Work out the finished part from the listing and answer in its coordinate system (mm). A direction names the side the tool comes from. Round coordinates to 2 decimals unless told otherwise and drop trailing zeros. Write each loop counter-clockwise with the first axis right and the second up, starting at its lowest first coordinate (ties: lowest second). Pieces come first, ordered by that corner, then holes. Notation, with made-up numbers: M 39.5,-28.75 L 51.5,-28.75 A17 cw 51.5,-13.75 Z; hole C 82,43 d4. An arc over 180 degrees is marked long. Answer in a Markdown table with one row per item.
Autodesk Inventor part; units mm, degrees
ref_plane "YZ Plane" through (0, 0, 0) normal (1, 0, 0) x (0, 1, 0)
ref_plane "XZ Plane" through (0, 0, 0) normal (0, 1, 0) x (-1, 0, 0)
ref_plane "XY Plane" through (0, 0, 0) normal (0, 0, 1) x (1, 0, 0)
sketch "Skizze1" plane through (0, 0, 0) normal (0, 1, 0) x (-1, 0, 0)
  line L0 (0, 0) -> (13.65, 0) construction
  line L1 (15.3, 9.35) -> (0, 9.35)
  line L2 (3.6, 5) -> (15.3, 5)
  line L3 (15.3, 5) -> (15.3, 9.35)
  line L4 (0, 9.35) -> (3.95, 9.35)
  line L5 (3.6, 5) -> (3.6, -5)
  line L6 (3.95, -9.35) -> (0, -9.35)
  line L7 (0, -9.35) -> (0, 9.35)
  line L8 (0, -9.35) -> (15.3, -9.35)
  line L9 (15.3, -9.35) -> (15.3, -5)
  line L10 (15.3, -5) -> (3.6, -5)
  dimension "d0" = 18.7
  dimension "d1" = 10
  dimension "d2" = 15.3
  dimension "d3" = 3.6
extrude "Extrusion1" add sketch "Skizze1" along normal blind 5
sketch "Skizze3" plane through (0, 0, 0) normal (1, 0, 0) x (0, 1, 0)
  line L0 (0, 9.35) -> (0, -9.35)
  line L1 (0, -9.35) -> (5, -9.35)
  line L2 (5, 9.35) -> (5, -9.35)
  line L3 (0, 9.35) -> (5, 9.35)
  line L4 (13.7, 10.15) -> (-1.55, 10.15)
  line L5 (-1.55, 10.15) -> (-1.55, -10.15)
  line L6 (-1.55, -10.15) -> (13.7, -10.15)
  line L7 (13.7, -10.15) -> (13.7, 10.15)
  line L8 (0, 0) -> (5, 0) construction
  dimension "d6" = 15.25
  dimension "d7" = 20.3
  dimension "d8" = 8.7
  dimension "d9" = 1.55
extrude "Extrusion2" add sketch "Skizze3" along normal blind 1.6 contours L3 L2 L1 L0 | L7 L6 L5 L4
chamfer "Fase1" distance 1 angle 45 2 edges at (-15.3, 0, -7.175) (-15.3, 0, 7.175)
properties part number "SYS IR Sensor"
1. Consider line 1 along X through (y, z) = (9.5, -6.25); line 2 along X through (y, z) = (1.5, -0.5); line 3 along Z through (x, y) = (-5, 3.75). Determine where each line is inside the solid, lowest interval first. Write a range as from..to.
Calculated:
| item | result |
|---|---|
| line 1 | x = 0..1.6 |
| line 2 | x = -3.6..1.6 |
| line 3 | z = -9.35..-5, 5..9.35 |
2. The part is cut by section B-B (z = -4.75). Determine the outline of the cut face in (x, y).
Calculated:
| item | result |
|---|---|
| outline | M -3.6,0 L 0,0 L 0,-1.55 L 1.6,-1.55 L 1.6,13.7 L 0,13.7 L 0,5 L -3.6,5 Z |
3. Given pin 1 (7 mm diameter, centred on x = -10, z = 4, fed in from -Y); pin 2 (1 mm diameter, centred on x = -8, z = -5, fed in from +Y); pin 3 (2 mm diameter, centred on x = -11.5, z = -2.5, fed in from -Y); pin 4 (7.5 mm diameter, centred on y = 3, z = -1.5, fed in from -X), each flat-ended and moving along its own axis, determine where each tip first touches the part or whether it passes through.
Calculated:
| item | result |
|---|---|
| pin 1 | stops at y = 0 |
| pin 2 | stops at y = 5 |
| pin 3 | passes through |
| pin 4 | stops at x = -15.3 |
4. The part is cut by section D-D (x = -1.5). Determine the outline of the cut face in (y, z).
Calculated:
| item | result |
|---|---|
| outline | M 0,-9.35 L 5,-9.35 L 5,9.35 L 0,9.35 Z |
5. Determine the mould class of faces 5 (the flat face through (-8, 2, -9.35)), 6 (the flat face through (-15.3, 3, -7)), 7 (the flat face through (-10, 2, -5)) for opening direction Z: released by +Z, released by -Z, zero draft, split by the parting line, or undercut.
Calculated:
| item | result |
|---|---|
| face 5 | released by -Z |
| face 6 | zero draft |
| face 7 | undercut |
6. The part is cut by section A-A (x = -10.5). Determine the outline of the cut face in (y, z).
Calculated:
| item | result |
|---|---|
| outline | M 0,-9.35 L 5,-9.35 L 5,-5 L 0,-5 Z; M 0,5 L 5,5 L 5,9.35 L 0,9.35 Z |
7. A tool of negligible diameter and unlimited length cuts with its end or side. For faces 1 (the flat face through (-8, 2, 9.35)), 2 (the flat face through (-2, 0, 0)), 3 (the flat face through (-2, 5, 0)), 4 (the flat face through (-9, 2, 5)), from which of +Z, -Z, +X, -X, +Y, -Y can it reach the whole face along a straight path? Write none if from no direction.
Calculated:
| item | result |
|---|---|
| face 1 | +Z, -X, +Y, -Y |
| face 2 | +Z, -Z, -X, -Y |
| face 3 | +Z, -Z, -X, +Y |
| face 4 | -X, +Y, -Y |
8. The part is cut by section C-C (y = 3). Determine the outline of the cut face in (x, z).
Calculated:
| item | result |
|---|---|
| outline | M -15.3,-9.35 L 0,-9.35 L 0,-10.15 L 1.6,-10.15 L 1.6,10.15 L 0,10.15 L 0,9.35 L -15.3,9.35 L -15.3,5 L -3.6,5 L -3.6,-5 L -15.3,-5 Z |
